Check sheet for the modelled part. Datum: model origin and axes. Units: mm. A direction names the side the tool comes from. Round coordinates to 2 decimals unless told otherwise and drop trailing zeros. Order: outer loops, then holes, each group sorted by start corner. A loop starts at its lowest first (then second) coordinate and runs counter-clockwise, first axis right, second up. Notation, with made-up numbers: (54.25, 68.5) -> (109.25, 68.5) arc R8 cw to (109.25, 75.5) -> close; hole circle Ø2 at (0.25, -7.5). An arc over 180 degrees is marked (long way). Answer in a Markdown table with one row per item.
```python
from build123d import *

# Parameters (mm, degrees)
SKIZZE1_R                       = 1.5
AUFSATZ_LINEAR_AUSTRAGEN1_DEPTH = 16
SCHNITT_LINEAR_AUSTRAGEN1_DEPTH = 2
SKIZZE3_R                       = 2.5
SCHNITT_LINEAR_AUSTRAGEN2_DEPTH = 7
SKIZZE4_R                       = 3.05
SCHNITT_LINEAR_AUSTRAGEN3_DEPTH = 2.1
VERRUNDUNG1_R                   = 1
SKIZZE5_R                       = 3.997213622
SCHNITT_LINEAR_AUSTRAGEN4_DEPTH = 28.540878708
SKIZZE6_W                       = 23.495930852
SKIZZE6_H                       = 2.64125978
SCHNITT_LINEAR_AUSTRAGEN5_DEPTH = 4


with BuildPart() as part:
    # Skizze1 → Aufsatz-Linear austragen1 (new body)
    with BuildSketch(Plane.XY):
        with BuildLine():
            Line((-16.1, 13.5), (16.1, 13.5))
            ThreePointArc((16.1, 13.5), (18.504163056, 12.504163056), (19.5, 10.1))
            Line((19.5, 10.1), (19.5, -10.1))
            ThreePointArc((19.5, -10.1), (18.504163056, -12.504163056), (16.1, -13.5))
            Line((16.1, -13.5), (-16.1, -13.5))
            ThreePointArc((-16.1, -13.5), (-18.504163056, -12.504163056), (-19.5, -10.1))
            Line((-19.5, -10.1), (-19.5, 10.1))
            ThreePointArc((-19.5, 10.1), (-18.504163056, 12.504163056), (-16.1, 13.5))
        make_face()
        with Locations((15, 8.5)):
            Circle(SKIZZE1_R, mode=Mode.SUBTRACT)
        with Locations((-15, -8.5)):
            Circle(SKIZZE1_R, mode=Mode.SUBTRACT)
    extrude(amount=AUFSATZ_LINEAR_AUSTRAGEN1_DEPTH)

    # Skizze2 → Schnitt-Linear austragen1 (cut)
    with BuildSketch(Plane.XY.offset(16)):
        with BuildLine():
            Line((-15, 4.5), (15, 4.5))
            ThreePointArc((15, 4.5), (16.414213562, 3.914213562), (17, 2.5))
            Line((17, 2.5), (17, -2.5))
            ThreePointArc((17, -2.5), (16.414213562, -3.914213562), (15, -4.5))
            Line((15, -4.5), (-15, -4.5))
            ThreePointArc((-15, -4.5), (-16.414213562, -3.914213562), (-17, -2.5))
            Line((-17, -2.5), (-17, 2.5))
            ThreePointArc((-17, 2.5), (-16.414213562, 3.914213562), (-15, 4.5))
        make_face()
    extrude(amount=-SCHNITT_LINEAR_AUSTRAGEN1_DEPTH, mode=Mode.SUBTRACT)

    # Skizze3 → Schnitt-Linear austragen2 (cut)
    with BuildSketch(Plane.XY.offset(14)):
        with Locations((-13, 0)):
            Circle(SKIZZE3_R)
        with Locations(Location((13, 0, 0), (0, 0, 180))):
            Circle(SKIZZE3_R)
    extrude(amount=-SCHNITT_LINEAR_AUSTRAGEN2_DEPTH, mode=Mode.SUBTRACT)

    # Skizze4 → Schnitt-Linear austragen3 (cut)
    with BuildSketch(Plane.XY.offset(16)):
        with Locations((15, 8.5)):
            Circle(SKIZZE4_R)
        with Locations((-15, -8.5)):
            Circle(SKIZZE4_R)
    extrude(amount=-SCHNITT_LINEAR_AUSTRAGEN3_DEPTH, mode=Mode.SUBTRACT)

    # Verrundung1
    verrundung1_edges = [part.edges().sort_by_distance(p)[0] for p in [
        (-18.504163056, 12.504163056, 16),
        (-19.5, 0, 16),
        (-18.504163056, -12.504163056, 16),
        (0, -13.5, 16),
        (18.504163056, -12.504163056, 16),
        (19.5, 0, 16),
        (18.504163056, 12.504163056, 16),
        (0, 13.5, 16),
    ]]
    fillet(verrundung1_edges, radius=VERRUNDUNG1_R)

    # Skizze5 → Schnitt-Linear austragen4 (cut, through all)
    with BuildSketch(Plane.XY.offset(14)):
        Circle(SKIZZE5_R)
    extrude(amount=-SCHNITT_LINEAR_AUSTRAGEN4_DEPTH, mode=Mode.SUBTRACT)

    # Skizze6 → Schnitt-Linear austragen5 (cut)
    with BuildSketch(Plane.XY.offset(14)):
        Rectangle(SKIZZE6_W, SKIZZE6_H)
    extrude(amount=-SCHNITT_LINEAR_AUSTRAGEN5_DEPTH, mode=Mode.SUBTRACT)


solid = part.part
```
(1) Tool access check on faces 4 (the cylindrical face through (19.215, -0.141, 15.699)), 5 (the flat face through (0, 4.5, 15)). Record the directions out of +Z, -Z, +X, -X, +Y, -Y that give a thin tool (end or side, any length) a straight path to the whole face; none if there is none.
Solutions:
| item | result |
|---|---|
| face 4 | +Z, +X, +Y, -Y |
| face 5 | +Z |
(2) Section check B-B on z = 9.5. Record the boundary of the cut face in (x, y), plus the area to 3 significant figures.
Solutions:
| item | result |
|---|---|
| outline | (-19.5, -10.1) arc R3.4 ccw to (-16.1, -13.5) -> (16.1, -13.5) arc R3.4 ccw to (19.5, -10.1) -> (19.5, 10.1) arc R3.4 ccw to (16.1, 13.5) -> (-16.1, 13.5) arc R3.4 ccw to (-19.5, 10.1) -> close; hole circle Ø3 at (-15, -8.5); hole circle Ø5 at (-13, 0); hole circle Ø7.99 at (0, 0); hole circle Ø5 at (13, 0); hole circle Ø3 at (15, 8.5) |
| area | 939 mm^2 |
(3) Section check C-C on y = 8.5. Record the boundary of the cut face in (x, z).
Solutions:
| item | result |
|---|---|
| outline | (-19.5, 0) -> (13.5, 0) -> (13.5, 13.9) -> (11.95, 13.9) -> (11.95, 16) -> (-18.5, 16) arc R1 ccw to (-19.5, 15) -> close; (16.5, 0) -> (19.5, 0) -> (19.5, 15) arc R1 ccw to (18.5, 16) -> (18.05, 16) -> (18.05, 13.9) -> (16.5, 13.9) -> close |
(4) Scan lines: probe 1 along Y at (x, z) = (0, 7.25); probe 2 along Y at (x, z) = (13, 11); probe 3 along Y at (x, z) = (15, 11). Record each from-to range of solid material in increasing order. Write a range as from..to.
Solutions:
| item | result |
|---|---|
| probe 1 | -13.5..-4, 4..13.5 |
| probe 2 | -13.5..-2.5, 2.5..13.5 |
| probe 3 | -13.5..-1.5, 1.5..7, 10..13.5 |
(5) Draft check along X on faces 1 (the cylindrical face through (-18.48, -12.53, 7.4)), 2 (the cylindrical face through (-0.225, -13.215, 15.699)), 3 (the cylindrical face through (-0.87, -3.9, 7.1)). Enter one of: pulls with the +X half, pulls with the -X half, needs draft (parallel to the pull), parting line crosses it, or undercut.
Solutions:
| item | result |
|---|---|
| face 1 | pulls with the -X half |
| face 2 | needs draft |
| face 3 | undercut |
(6) Depth check by flat-ended pin: pin 1 Ø0.6 at (x, z) = (6, 15.5) entering from -Y; pin 2 Ø4 at (x, y) = (2.5, -9.5) entering from -Z; pin 3 Ø4 at (x, y) = (-13, 0) entering from +Z; pin 4 Ø4.5 at (x, y) = (6, 1) entering from +Z. Enter the tip coordinate at first touch or a pass-through.
Solutions:
| item | result |
|---|---|
| pin 1 | y = -13.48 |
| pin 2 | z = 0 |
| pin 3 | z = 7 |
| pin 4 | z = 14 |
(7) Section check A-A on x = 0. Record the boundary of the cut face in (y, z).
Solutions:
| item | result |
|---|---|
| outline | (-13.5, 0) -> (-4, 0) -> (-4, 14) -> (-4.5, 14) -> (-4.5, 16) -> (-12.5, 16) arc R1 ccw to (-13.5, 15) -> close; (4, 0) -> (13.5, 0) -> (13.5, 15) arc R1 ccw to (12.5, 16) -> (4.5, 16) -> (4.5, 14) -> (4, 14) -> close |
(8) Section check D-D on x = 12.5. Record the boundary of the cut face in (y, z), plus the area to 3 significant figures.
Solutions:
| item | result |
|---|---|
| outline | (-13.5, 0) -> (13.5, 0) -> (13.5, 15) arc R1 ccw to (12.5, 16) -> (10.25, 16) -> (10.25, 13.9) -> (6.75, 13.9) -> (6.75, 16) -> (4.5, 16) -> (4.5, 14) -> (2.45, 14) -> (2.45, 7) -> (-2.45, 7) -> (-2.45, 14) -> (-4.5, 14) -> (-4.5, 16) -> (-12.5, 16) arc R1 ccw to (-13.5, 15) -> close |
| area | 372 mm^2 |
